```python
from build123d import *

# Parameters (mm, degrees)
F1_DEPTH     = 76.2
F2_SIZE      = 5.08
F4_DEPTH     = 152.4
F5_R         = 50.4680515056
F6_DEPTH     = 76.2
F7_R         = 22.662684834
F8_DEPTH     = 228.6
F9_R         = 5.08
F10_T1_DEPTH = 217.1500590573
F10_T3_DEPTH = 210.0843614146
F10_T5_DEPTH = 180.2491648874


# Not quite as in the source:
# - a fillet or chamfer that OpenCascade refuses, or shapes differently, is made with other operations: its cross-section is extruded or revolved along the edge and cut away or added


with BuildPart() as f1:
    # F0 (on Front) → F1 (new body)
    with BuildSketch(Plane.XZ):
        Polygon((376.9832551479, 180.0154298544), (-138.5454237461, 237.0085567236), (-306.9341778755, 20.6937491894), (13.0044706166, -207.2787433863), (317.3995614052, -115.3125613928), (376.9832551479, 16.8078560382), align=None)
    extrude(amount=F1_DEPTH)

    # F2
    f2_edges = [f1.edges().sort_by_distance(p)[0] for p in [
        (-146.964854, -76.2, -93.292497),
        (165.202016, -76.2, -161.295652),
        (347.191408, -76.2, -49.252353),
        (376.983255, -76.2, 98.411643),
        (119.218916, -76.2, 208.511993),
        (-222.739801, -76.2, 128.851153),
    ]]
    chamfer(f2_edges, length=F2_SIZE)

    # F3 (on face) → F4 (join)
    with BuildSketch(Plane.XZ.offset(76.2)):
        Polygon((132.2494894266, 45.2478192747), (16.2920933217, 102.7888357639), (0, -55.6601323187), align=None)
    extrude(amount=F4_DEPTH)

    # F5 (on face) → F6 (cut)
    with BuildSketch(Plane.XZ.offset(76.2)):
        with Locations((-138.9218121767, 108.8546961546)):
            Circle(F5_R)
    extrude(amount=-F6_DEPTH, mode=Mode.SUBTRACT)

    # F7 (on face) → F8 (cut)
    with BuildSketch(Plane.XZ.offset(228.6)):
        with Locations((51.4107942581, 38.0054563284)):
            Circle(F7_R)
    extrude(amount=-F8_DEPTH, mode=Mode.SUBTRACT)

    # F9
    f9_edges = [f1.edges().sort_by_distance(p)[0] for p in [
        (-146.964854, 0, -93.292497),
        (165.202016, 0, -161.295652),
        (347.191408, 0, -49.252353),
        (376.983255, 0, 98.411643),
        (119.218916, 0, 208.511993),
        (-222.739801, 0, 128.851153),
    ]]
    fillet(f9_edges, radius=F9_R)

    # F10: fillet of radius 10.16 on 4 edges, made by hand

    # F10_s2 → F10_t1 (cut)
    with BuildSketch(Plane(origin=(-47.0353574765, 0, -35.8885436609), x_dir=(0, 1, 0), z_dir=(0.7950071685, 0, 0.6066000347))):
        with BuildLine():
            ThreePointArc((-218.44, -44.2502041916), (-225.6242048969, -41.2744090884), (-228.6, -34.0902041916))
            Line((-228.6, -34.0902041916), (-228.6, -44.2502041916))
            Line((-228.6, -44.2502041916), (-218.44, -44.2502041916))
        make_face()
    extrude(amount=F10_T1_DEPTH, mode=Mode.SUBTRACT)

    # F10_s4 → F10_t3 (cut)
    with BuildSketch(Plane(origin=(13.2268524744, 0, 128.6379278687), x_dir=(0, 1, 0), z_dir=(-0.102283069, 0, -0.9947553336))):
        with BuildLine():
            ThreePointArc((-218.44, 5.6930891519), (-225.6242048969, 8.668884255), (-228.6, 15.8530891519))
            Line((-228.6, 15.8530891519), (-228.6, 5.6930891519))
            Line((-228.6, 5.6930891519), (-218.44, 5.6930891519))
        make_face()
    extrude(amount=F10_T3_DEPTH, mode=Mode.SUBTRACT)

    # F10_s6 → F10_t5 (cut)
    with BuildSketch(Plane(origin=(110.8548223357, 0, -55.0089892857), x_dir=(0, 1, 0), z_dir=(-0.8957755441, 0, 0.4445066644))):
        with BuildLine():
            ThreePointArc((-218.44, -99.3176693375), (-225.6242048969, -96.3418742344), (-228.6, -89.1576693375))
            Line((-228.6, -89.1576693375), (-228.6, -99.3176693375))
            Line((-228.6, -99.3176693375), (-218.44, -99.3176693375))
        make_face()
    extrude(amount=F10_T5_DEPTH, mode=Mode.SUBTRACT)

    # F10_s7 → F10_t8 (revolve, cut)
    with BuildSketch(Plane.XY.offset(38.0054563284)):
        with BuildLine():
            ThreePointArc((74.0734790921, -218.44), (77.0492741953, -225.6242048969), (84.2334790921, -228.6))
            Line((84.2334790921, -228.6), (74.0734790921, -228.6))
            Line((74.0734790921, -228.6), (74.0734790921, -218.44))
        make_face()
    revolve(axis=Axis((51.4107942581, -228.6, 38.0054563284), (0, -1, 0)), mode=Mode.SUBTRACT)


solid = f1.part
```
Geometry: final body of the model. Coordinates: model frame, mm. A direction names the side the tool comes from. Round coordinates to 2 decimals unless told otherwise and drop trailing zeros. Order: outer loops, then holes, each group sorted by start corner. A loop starts at its lowest first (then second) coordinate and runs counter-clockwise, first axis right, second up. Notation, with made-up numbers: (74.25, 32) -> (93.25, 32) arc R29 ccw to (93.25, 66) -> close; hole circle Ø4 at (50, -26). An arc over 180 degrees is marked (long way). Use one line per item in the form item = value. Start each with the question number.
1. Pin query (flat end, axial travel): pin 1 Ø6 at (x, z) = (22.5, -162.5) entering from -Y; pin 2 Ø5 at (y, z) = (-72.5, -41.5) entering from +X; pin 3 Ø2 at (y, z) = (-69, 170) entering from -X. Return the tip coordinate at first contact, or that it passes through.
2. Cut plane B-B (y = -119). Return the cut outline in (x, z), then the cut area to 3 significant figures.
3. Reachability of faces 1 (the face through (51, -228.6, 5)), 2 (the face through (75.082, -146.324, 73.616)) from +Z, -Z, +X, -X, +Y, -Y: full face, straight path, thin tool, end or side. Return the list, or none.
4. Draft query along Z for faces 3 (the face through (376.983, -38, 97)), 4 (the face through (-221.561, -37.638, 130.365)), 5 (the face through (346.774, -37.638, -50.177)), 6 (the face through (72.345, -110.749, 29.326)). Return one class per face: pulls with the +Z half, pulls with the -Z half, needs draft (parallel to the pull), parting line crosses it, or undercut.
5. Line query: probe 1 along Y at (x, z) = (202, -136); probe 2 along Z at (x, y) = (60, -205); probe 3 along Z at (x, y) = (39.5, -167). Output: solid intervals per line, ascending.
6. Cut plane A-A (y = -22). Return the cut outline in (x, z), then the cut area to 3 significant figures.
Solution:
q1.pin_1 = -76.2
q1.pin_2 = 351.63
q1.pin_3 = -191.49
q2.outline = (0, -55.66) -> (132.25, 45.25) -> (16.29, 102.79) -> close; hole circle Ø45.33 at (51.41, 38.01)
q2.area = 8,040 mm^2
q3.face_1 = +Z, -Z, +X, -X, -Y
q3.face_2 = +Z, +X, -Y
q4.face_3 = needs draft
q4.face_4 = pulls with the +Z half
q4.face_5 = pulls with the -Z half
q4.face_6 = undercut
q5.probe_1 = -76.2 to 0
q5.probe_2 = -9.88 to 17.03, 58.98 to 81.1
q5.probe_3 = -25.52 to 18.73, 57.29 to 91.27
q6.outline = (-306.93, 20.69) -> (13, -207.28) -> (317.4, -115.31) -> (376.98, 16.81) -> (376.98, 180.02) -> (-138.55, 237.01) -> close; hole circle Ø100.94 at (-138.92, 108.85); hole circle Ø45.33 at (51.41, 38.01)
q6.area = 201,000 mm^2
